Geometry: final body of the model. Coordinates: model frame, mm. A direction names the side the tool comes from. Coordinates: 2 decimals unless noted, no trailing zeros. Write each loop counter-clockwise with the first axis right and the second up, starting at its lowest first coordinate (ties: lowest second). Pieces come first, ordered by that corner, then holes. Notation, with made-up numbers: (23.25, 29) -> (56.25, 29) arc R20 cw to (56.25, 54) -> close; hole circle Ø11 at (-20, 82.25). An arc over 180 degrees is marked (long way). One line per item, written item: value. Start each with the question number.
Autodesk Inventor part; units mm, degrees
ref_plane "Work Plane1" through (1.525, 0, 0) normal (0, 0, 1) x (1, 0, 0)
ref_plane "YZ Plane" through (0, 0, 0) normal (1, 0, 0) x (0, 1, 0)
ref_plane "XZ Plane" through (0, 0, 0) normal (0, 1, 0) x (-1, 0, 0)
sketch "Sketch1" plane through (0, 0, 0) normal (0, 0, 1) x (1, 0, 0)
  line L0 (0, 7.315) -> (0, 5)
  line L1 (4.5, 5) -> (35, 5)
  line L2 (35, 5) -> (35, 0)
  line L3 (35, 0) -> (-0.6001, 0)
  line L4 (-7.7201, 0) -> (42.12, 0)
  line L5 (-0.6001, 0) -> (-0.6001, 7.315)
  line L6 (-0.6001, 7.315) -> (0, 7.315)
  line L7 (4.5, 5) -> (3.5797, 5)
  line L8 (3.5797, 5) -> (0, 5)
  line L9 (0, -1.463) -> (0, 8.778)
  dimension "d0" = 35
  dimension "d1" = 30.5
  dimension "d2" = 10
  dimension "d9" = 0.6001
  dimension "d10" = 14.63
  dimension "d13" = 0.9203
  dimension "d14" = 10
revolve "Body" add sketch "Sketch1" angle 360 about axis through (35, 0, 0) along (-1, 0, 0)
sketch "Sketch2" plane through (-0.6001, 0, 0) normal (-1, 0, 0) x (0, 0, 1)
  line L0 (0, 9.2376) -> (8, 4.6188)
  line L1 (8, 4.6188) -> (8, -4.6188)
  line L2 (8, -4.6188) -> (0, -9.2376)
  line L3 (0, -9.2376) -> (-8, -4.6188)
  line L4 (-8, -4.6188) -> (-8, 4.6188)
  line L5 (-8, 4.6188) -> (0, 9.2376)
  point P0 (0, 0)
  point P1 (0, 0)
  dimension "d11" = 16
extrude "Head" add sketch "Sketch2" along normal blind 5.8
sketch "Sketch4" plane through (0, 0, 0) normal (0, 0, 1) x (1, 0, 0)
  line L0 (-6.4001, 8) -> (-6.4001, 9.2376)
  line L1 (-6.4001, 9.2376) -> (-5.6856, 9.2376)
  line L2 (-5.6856, 9.2376) -> (-6.4001, 8)
  line L3 (-7.5601, 0) -> (0.5599, 0)
  line L4 (-0.6001, 9.2376) -> (-6.4001, 9.2376)
  line L5 (-6.4001, 4.6188) -> (-6.4001, 9.2376)
  dimension "d5" = 30
  dimension "d19" = 16
revolve "Chamfer1" cut sketch "Sketch4" angle 360 about axis through (-10, 0, 0) along (1, 0, 0)
thread "Thread"
chamfer "Chamfer2" distance 0.9202 distance2 0.9203 1 edges at (35, -5, 0) measured on face at (35, -0.8768, 0.3989)
ref_plane "Work Plane1" through (1.525, 0, 0) normal (0, 0, 1) x (1, 0, 0)
equation "\"d11\" = SW"
equation "\"d3\" = KOH - SD"
equation "\"d15\" = GEL"
equation "\"d6\" = -0.5 * SPD + 0.5 * GD"
equation "\"d0\" = NLG"
equation "\"d1\" = GEL"
equation "\"d2\" = GD"
equation "\"d10\" = SD2"
equation "\"d14\" = BDM"
equation "\"d5\" = ANG1"
equation "\"d19\" = SW0"
equation "\"NLG\" = 35"
equation "\"GD\" = NND"
equation "\"BDM\" = NND"
equation "\"KOH\" = 6.4"
equation "\"GEL\" = 30.5"
equation "\"SW\" = 16"
equation "\"SW0\" = SW"
equation "\"SPD\" = NND - 1.2269 * PTC"
equation "\"SD2\" = 14.63"
equation "\"SD\" = 0.6"
equation "\"ANG1\" = 30deg"
equation "\"GAL\" = 0.61345 * PTC"
equation "\"GUL\" = 0.61345 * PTC"
equation "\"RR\" = 0.4"
equation "\"GD1\" = THREADDIA - 1.2269 * PTC"
equation "\"SDH\" = SD2"
equation "\"SDHG\" = 4.5"
equation "\"TOA\" = 30deg"
equation "\"PTC\" = 1.5"
equation "\"E0\" = 18.48"
properties part number "ISO 4017 - M10 x 35" material "Steel, Mild"
Q1. Line query: L1, parallel to X at y = 4, z = 5; L2, parallel to Y at x = 26, z = -3; L3, parallel to X at y = -7, z = 2.25. Output: solid intervals per line, ascending. Write a range as from..to.
Q2. Cut plane A-A on x = 30. Output: boundary loops of the cut face in (y, z), and give its area (3 significant figures).
Q3. Access query for faces 1 (the flat face through (-0.6, -7, -3)), 2 (the flat face through (-3.46, -6.896, 4.056)). Directions: +Z, -Z, +X, -X, +Y, -Y. A direction counts if a zero-diameter tool reaches every point of the face in a straight line with its end or side. Return the directions, or none.
Q4. First-contact query: P1, Ø4, axis at x = 30.5, y = -2, coming from the +Z side; P2, Ø3, axis at x = 27, z = -3.5, coming from the +Y side; P3, Ø2, axis at x = 22, z = 0.5, coming from the +Y side. Flat tips, straight axial feed; report the tip coordinate or a pass-through.
Solution:
1. L1: -6.4..0
1. L2: -4..4
1. L3: -6.4..-0.6
2. outline: circle Ø10 at (0, 0)
2. area: 78.5 mm²
3. face 1: +X
3. face 2: +Z, +X, -X, -Y
4. P1: z = 5
4. P2: y = 4.58
4. P3: y = 5
